The listing builds one solid part. Answer for the finished solid, in the listing's coordinates (mm). Face numbers are marked on the shaded views. A direction names the side the tool comes from. Give positions to 0.01 mm unless a question says otherwise; leave off trailing zeros. Write each loop counter-clockwise with the first axis right and the second up, starting at its lowest first coordinate (ties: lowest second). Pieces come first, ordered by that corner, then holes. Notation, with made-up numbers: (-34, 60) - (-4, 60) arc R21 ccw to (-4, 79) - close; hole circle Ø11 at (21, 59.5). An arc over 180 degrees is marked (long way). Return JSON: item names as keys, results as strings.
from build123d import *

# Parameters (mm, degrees)
CROQUIS3_W              = 50
CROQUIS3_H              = 30
VACIADO1_T              = -4
CORTAR_EXTRUIR1_REACH   = 78.811
CROQUIS7_R              = 12
REDONDEO1_R             = 5
SALIENTE_EXTRUIR1_DEPTH = 4
MATRIZC10_COUNT         = 4


with BuildPart() as part:
    # Croquis3 → Revolución1 (revolve)
    with BuildSketch(Plane(origin=(0, 0, 0), x_dir=(0, 0, -1), z_dir=(1, 0, 0)), mode=Mode.PRIVATE) as revoluci_n1_sk:
        with Locations((-25, 15)):
            Rectangle(CROQUIS3_W, CROQUIS3_H)
    revolve(revoluci_n1_sk.sketch.rotate(Axis((0, 0, 0), (0, 1, 0)), 180), axis=Axis((0, 0, 0), (0, 1, 0)))

    # Croquis6 → Cortar-Revolución1 (revolve, cut)
    with BuildSketch(Plane.XY, mode=Mode.PRIVATE) as cortar_revoluci_n1_sk:
        Polygon((-50, 30), (-50, 0), (-41.961524227, 30), align=None)
    revolve(cortar_revoluci_n1_sk.sketch.rotate(Axis((0, -970, 0), (0, 1, 0)), 180), axis=Axis((0, -970, 0), (0, 1, 0)), mode=Mode.SUBTRACT)

    # Vaciado1
    vaciado1_openings = [part.faces().sort_by_distance(p)[0] for p in [
        (0, 0, 0),
    ]]
    offset(amount=VACIADO1_T, openings=vaciado1_openings, kind=Kind.INTERSECTION)

    # Croquis7 → Cortar-Extruir1 (cut, up to next)
    with BuildSketch(Plane(origin=(0, 30, 0), x_dir=(1, 0, 0), z_dir=(0, 1, 0)), mode=Mode.PRIVATE) as cortar_extruir1_sk1:
        with Locations(Location((0, 0, 0), (0, 0, 270))):
            Circle(CROQUIS7_R)
    cortar_extruir1_tool1 = extrude(cortar_extruir1_sk1.sketch, amount=-CORTAR_EXTRUIR1_REACH, mode=Mode.PRIVATE) & part.part
    add(cortar_extruir1_tool1.solids().sort_by_distance((0, 30, 0))[0], mode=Mode.SUBTRACT)

    # Redondeo1
    redondeo1_edges = [part.edges().sort_by_distance(p)[0] for p in [
        (-41.961524227, 30, 0),
    ]]
    fillet(redondeo1_edges, radius=REDONDEO1_R)

    # Croquis8 → Saliente-Extruir1 (add)
    with BuildSketch(Plane(origin=(0, 0, 0), x_dir=(-1, 0, 0), z_dir=(0, -1, 0))):
        Polygon((0, 57.899543771), (5, 57.899543771), (10, 45.858895278), (0, 45.858895278), align=None)
    saliente_extruir1 = extrude(amount=-SALIENTE_EXTRUIR1_DEPTH)

    # Simetría1: Saliente-Extruir1 across plane
    add(saliente_extruir1.mirror(Plane(origin=(0, 4, -45.858895278), x_dir=(0, 0, 1), z_dir=(1, 0, 0))))

    # MatrizC10: Saliente-Extruir1 ×4 about axis
    matrizc10_axis = Axis((0, 0, 0), (0, 1, 0))
    for i in range(1, MATRIZC10_COUNT):
        add(saliente_extruir1.rotate(matrizc10_axis, i * 360 / MATRIZC10_COUNT))


solid = part.part
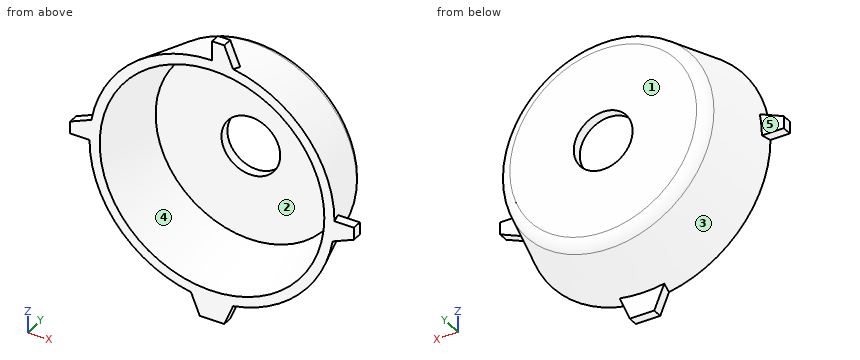
Item 1: Flat-ended cylindrical pins translate along their axes: P1, Ø10, axis at y = 15, z = 9.5, coming from the +X side; P2, Ø2.5, axis at x = 54.5, z = -5.5, coming from the +Y side; P3, Ø4, axis at y = 23, z = 38.5, coming from the +X side; P4, Ø6, axis at x = -4, y = 6, coming from the -Z side. Find the tip coordinate at first contact, or state that the pin passes through.
Answer below:
{"P1": "stops at x = 46.62", "P2": "stops at y = 4", "P3": "stops at x = 24.43", "P4": "stops at z = -57.9"}
Item 2: For the marked faces 1 and 2, determine the directions among +Z, -Z, +X, -X, +Y, -Y from which every point of the face is accessible in a straight line to the end or side of a thin tool.
Answer below:
{"face 1": "+Z, -Z, +X, -X, +Y", "face 2": "-Y"}
Item 3: A cutting plane is placed at A-A on y = 2. Determine the outline of the cut face in (x, z), then the cut area to 3 significant figures.
Answer below:
{"outline": "(-57.9, 0) - (-49.46, 0) arc R49.46 ccw to (-8.83, -48.67) - (-5, -57.9) - (5, -57.9) - (8.83, -48.67) arc R49.46 ccw to (48.67, -8.83) - (57.9, -5) - (57.9, 0) - (49.46, 0) arc R49.46 ccw to (8.83, 48.67) - (5, 57.9) - (0, 57.9) - (0, 49.46) arc R49.46 ccw to (-48.67, 8.83) - (-57.9, 5) - close; hole circle Ø90.65 at (0, 0)", "area": "1,530 mm²"}
Item 4: A cutting plane is placed at B-B on y = 16.5. Determine the outline of the cut face in (x, z).
Answer below:
{"outline": "circle Ø91.16 at (0, 0); hole circle Ø82.88 at (0, 0)"}
Item 5: The mould has two halves that part along Z. Classify the marked faces 3, 4 and 5: +Z half, -Z half, draft (parallel to the pull), parting line (faces both ways), or undercut.
Answer below:
{"face 3": "parting line", "face 4": "undercut", "face 5": "draft"}
Item 6: A cutting plane is placed at C-C on y = 10.5. Determine the outline of the cut face in (x, z).
Answer below:
{"outline": "circle Ø94.37 at (0, 0); hole circle Ø86.09 at (0, 0)"}
Item 7: Consider L1, parallel to Y at x = -10, z = -20; L2, parallel to X at y = 29, z = -4; L3, parallel to X at y = 20.5, z = -2. Determine where each line is inside the solid, lowest interval first.
Answer below:
{"L1": "y = 26 to 30", "L2": "x = -40.93 to -11.31, 11.31 to 40.93", "L3": "x = -44.46 to -40.32, 40.32 to 44.46"}
